Input: dimensioned drawing with shaded views. Units: mm. Origin: part minimum x, y, z. Coordinates: 2 decimals unless noted, no trailing zeros. Order: outer loops, then holes, each group sorted by start corner. A loop starts at its lowest first (then second) coordinate and runs counter-clockwise, first axis right, second up. Notation, with made-up numbers: (44.5, -34.5) - (55.5, -34.5) arc R38 ccw to (55.5, 4.5) - close; hole circle Ø4 at (62.25, 17). An arc over 180 degrees is marked (long way). Answer as CSV lines item,"result". Start each with the question number.
Item 1: First-contact query: pin 1 (1.5 mm diameter, centred on x = 281, y = 2.5, fed in from -Z); pin 2 (5.5 mm diameter, centred on x = 84.57, z = 25.43, fed in from +Y); pin 3 (1.5 mm diameter, centred on y = 3.5, z = 290, fed in from -X); pin 4 (1.5 mm diameter, centred on x = 12, y = 3.5, fed in from +Z). Flat tips, straight axial feed; report the tip coordinate or a pass-through.
Item 2: Section A-A (y = 2.2). Output: boundary loops of the cut face in (x, z), and give its area (3 significant figures).
Item 3: Material intervals for line 1 along X through (y, z) = (2.95, 25.43); line 2 along Z through (x, y) = (14.5, 0.7), sorted ascending.
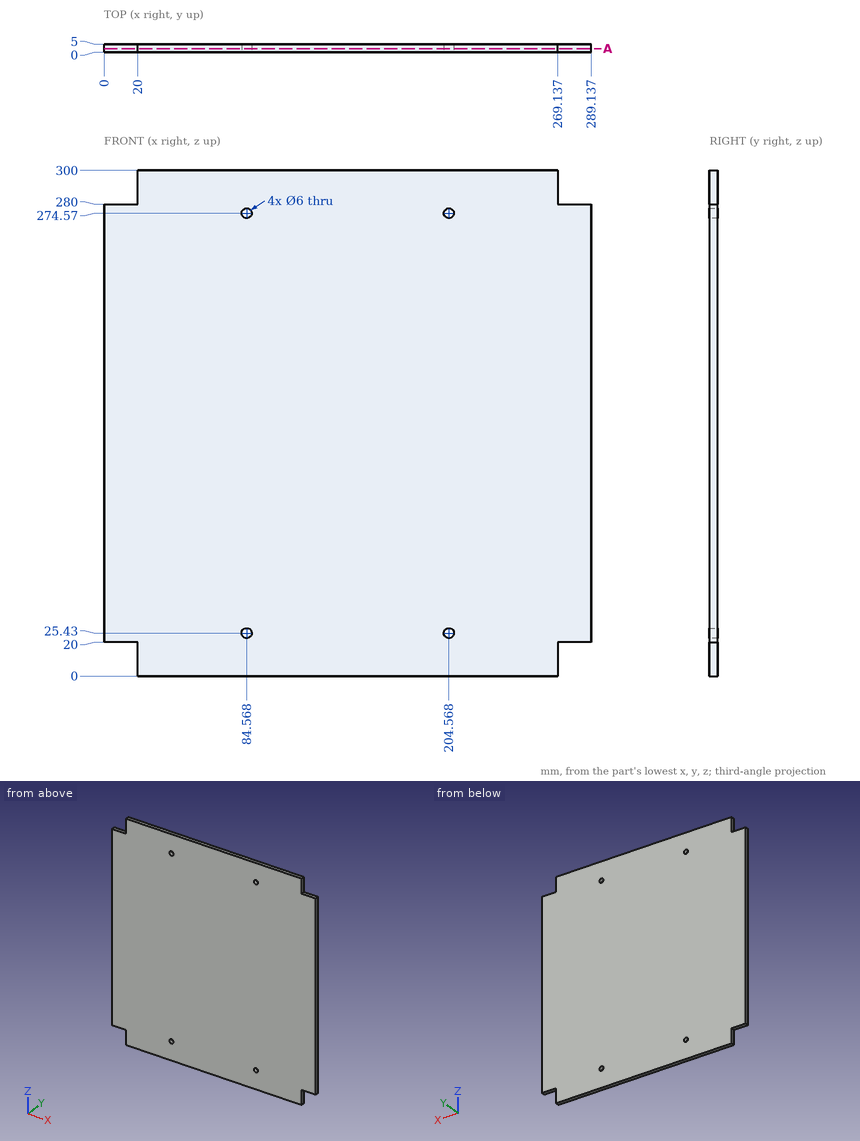
Determined:
1,pin 1,"stops at z = 20"
1,pin 2,"passes through"
1,pin 3,"stops at x = 20"
1,pin 4,"stops at z = 280"
2,outline,"(0, 20) - (20, 20) - (20, 0) - (269.14, 0) - (269.14, 20) - (289.14, 20) - (289.14, 280) - (269.14, 280) - (269.14, 300) - (20, 300) - (20, 280) - (0, 280) - close; hole circle Ø6 at (84.57, 25.43); hole circle Ø6 at (84.57, 274.57); hole circle Ø6 at (204.57, 25.43); hole circle Ø6 at (204.57, 274.57)"
2,area,"85,000 mm^2"
3,line 1,"x = 0 to 81.57, 87.57 to 201.57, 207.57 to 289.14"
3,line 2,"z = 20 to 280"
